Answer from the drawing. Dimensions are ordinates in mm from the lowest x, y and z of the part. A direction names the side the tool comes from. Give positions to 0.01 mm unless a question says otherwise; leave off trailing zeros. Write each loop counter-clockwise with the first axis right and the second up, starting at its lowest first coordinate (ties: lowest second). Pieces come first, ordered by that corner, then holes.
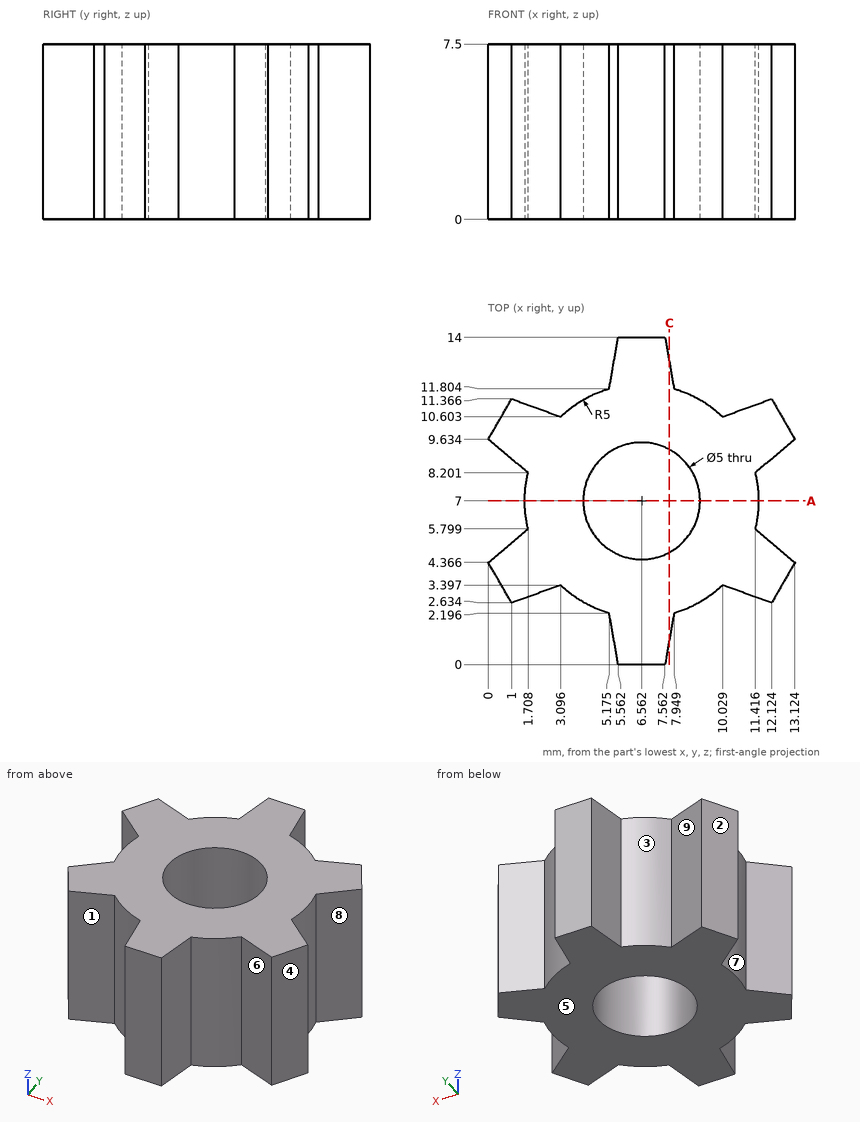
Item 1: Which of the six approach directions +Z, -Z, +X, -X, +Y, -Y give full straight-line access (tool end or side, diameter ignored) to the marked faces 5, 6, 7, 8 and 9?
Result set:
face 5: -Z, +X, -X, +Y, -Y
face 6: +Z, -Z, -Y
face 7: +Z, -Z, -X
face 8: +Z, -Z, +X
face 9: +Z, -Z, +Y
Item 2: Determine the mould class of the marked faces 1, 2, 3 and 4 for opening direction X: pulls with the +X half, pulls with the -X half, needs draft (parallel to the pull), parting line crosses it, or undercut.
Result set:
face 1: undercut
face 2: pulls with the -X half
face 3: undercut
face 4: pulls with the +X half
Item 3: Section C-C (x = 7.75) is taken. Write down the section's boundary in (y, z) (1 decimal).
Result set:
outline: (1.1, 0) - (4.8, 0) - (4.8, 7.5) - (1.1, 7.5) - close; (9.2, 0) - (12.9, 0) - (12.9, 7.5) - (9.2, 7.5) - close
Item 4: Each of these flat-tipped pins is pushed along its axis until it touches: pin 1 Ø6.5 at (x, y) = (6.56, 7) entering from +Z; pin 2 Ø1.5 at (y, z) = (8, 3) entering from -X (1 decimal); pin 3 Ø2 at (y, z) = (12.5, 6.5) entering from +X (1 decimal); pin 4 Ø3 at (x, z) = (11.5, 3) entering from +Y. Where does it stop, or does it pass through?
Result set:
pin 1: stops at z = 7.5
pin 2: stops at x = 1.1
pin 3: stops at x = 8.7
pin 4: stops at y = 11.37
Item 5: Section A-A (y = 7) is taken. Write down the section's boundary in (x, z).
Result set:
outline: (1.56, 0) - (4.06, 0) - (4.06, 7.5) - (1.56, 7.5) - close; (9.06, 0) - (11.56, 0) - (11.56, 7.5) - (9.06, 7.5) - close
Item 6: Find the intervals of material crossed by line 1 along Y through (x, z) = (6.5, 6.5); line 2 along Y through (x, z) = (6, 3.5) (1 decimal); line 3 along X through (y, z) = (5, 7.25) (1 decimal), in increasing order.
Result set:
line 1: y = 0 to 4.5, 9.5 to 14
line 2: y = 0 to 4.6, 9.4 to 14
line 3: x = 0.8 to 5.1, 8.1 to 12.4
